Geometry check sheet. Reference: the model listing, model coordinates, mm. Face numbers are marked on the shaded views. A direction names the side the tool comes from. Round coordinates to 2 decimals unless told otherwise and drop trailing zeros. Order: outer loops, then holes, each group sorted by start corner. A loop starts at its lowest first (then second) coordinate and runs counter-clockwise, first axis right, second up.
(1) Material ranges on line 1 along Y through (x, z) = (16.5, 0.9); line 2 along Y through (x, z) = (-15.5, 0.25); line 3 along Z through (x, y) = (-14.5, 12), recorded low to high.
(2) Sectioned sample at A-A (z = -2.75). Record the boundary of the cut face in (x, y).
(3) Go/stop test with flat-tipped pins: pin 1 (2 mm diameter, centred on y = -2, z = -2.5, fed in from -X); pin 2 (1 mm diameter, centred on y = 1, z = -1, fed in from +X); pin 3 (1.2 mm diameter, centred on x = 19, z = -4, fed in from +Y). Record where each tip stops, or that it passes through.
(4) Sectioned sample at C-C (y = 9.4). Record the boundary of the cut face in (x, z).
(5) Release check for a two-part mould opening along X. For the marked faces 1 and 2 record: +X half, -X half, draft (parallel to the pull), parting line (faces both ways), or undercut.
(6) Set-up check for the marked faces 3 and 4: record each of +Z, -Z, +X, -X, +Y, -Y from which the full face is reachable in a straight line by a thin tool's end or side.
(7) Sectioned sample at B-B (x = 16.5). Record the boundary of the cut face in (y, z), plus the area to 4 significant figures.
(8) Sectioned sample at D-D (x = 4.5). Record the boundary of the cut face in (y, z).
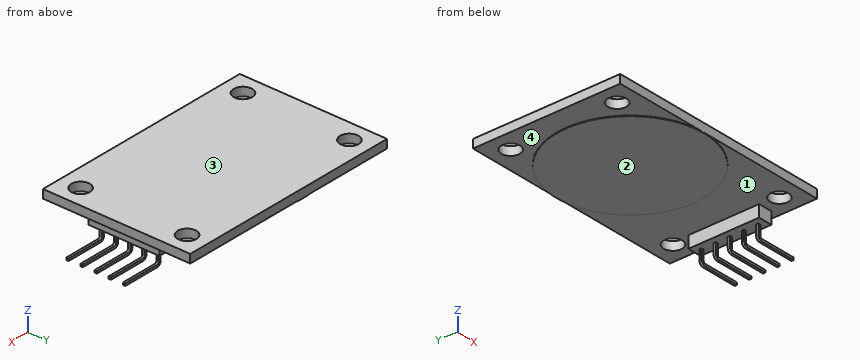
from build123d import *

# Parameters (mm, degrees)
SKETCH_1_W          = 40
SKETCH_1_H          = 26
EXTRUDE_1_DEPTH     = 1.5
SKETCH_2_R          = 1.65
CUT_EXTRUDE_1_DEPTH = 1.5
SKETCH_3_R          = 13
EXTRUDE_2_DEPTH     = 0.1
SKETCH_4_W          = 2.5
SKETCH_4_H          = 12.5
EXTRUDE_3_DEPTH     = 2.1
SKETCH_5_W          = 0.4
SKETCH_5_H          = 0.4


with BuildPart() as part:
    # 草图1 → 凸台-拉伸1 (new body)
    with BuildSketch(Plane.XY):
        Rectangle(SKETCH_1_W, SKETCH_1_H)
    extrude(amount=EXTRUDE_1_DEPTH)

    # 草图2 → 切除-拉伸1 (cut)
    with BuildSketch(Plane.XY.offset(1.5)):
        with Locations((-16.5, 9.4)):
            Circle(SKETCH_2_R)
        with Locations((16.5, 9.4)):
            Circle(SKETCH_2_R)
        with Locations((16.5, -9.4)):
            Circle(SKETCH_2_R)
        with Locations((-16.5, -9.4)):
            Circle(SKETCH_2_R)
    extrude(amount=-CUT_EXTRUDE_1_DEPTH, mode=Mode.SUBTRACT)

    # 草图3 → 凸台-拉伸2 (add)
    with BuildSketch(Plane(origin=(0, 0, 0), x_dir=(-1, 0, 0), z_dir=(0, 0, -1))):
        with Locations(Location((3, 0, 0), (0, 0, 270))):
            Circle(SKETCH_3_R)
    extrude(amount=EXTRUDE_2_DEPTH)

    # 草图4 → 凸台-拉伸3 (add)
    with BuildSketch(Plane(origin=(0, 0, 0), x_dir=(-1, 0, 0), z_dir=(0, 0, -1))):
        with Locations((-17.25, 0)):
            Rectangle(SKETCH_4_W, SKETCH_4_H)
    extrude(amount=EXTRUDE_3_DEPTH)

    # 扫描1: sweep along a path in 草图6
    with BuildLine(Plane(origin=(0, 5.2, 0), x_dir=(-1, 0, 0), z_dir=(0, -1, 0))) as sweep_1_path:
        Line((-17.25, 2.1), (-17.25, 3.9))
        ThreePointArc((-17.25, 3.9), (-17.396446609, 4.253553391), (-17.75, 4.4))
        Line((-17.75, 4.4), (-24.25, 4.4))
    # 草图5 → 扫描1 (sweep)
    with BuildSketch(Plane(origin=(0, 0, -2.1), x_dir=(-1, 0, 0), z_dir=(0, 0, -1))):
        with Locations((-17.25, 2.5)):
            Rectangle(SKETCH_5_W, SKETCH_5_H)
        with Locations((-17.25, 5)):
            Rectangle(SKETCH_5_W, SKETCH_5_H)
        with Locations((-17.25, 0)):
            Rectangle(SKETCH_5_W, SKETCH_5_H)
        with Locations((-17.25, -2.5)):
            Rectangle(SKETCH_5_W, SKETCH_5_H)
        with Locations((-17.25, -5)):
            Rectangle(SKETCH_5_W, SKETCH_5_H)
    sweep(path=sweep_1_path.line)


solid = part.part
Answer below:
1. line 1: y = -13 to -11.05, -7.75 to 7.75, 11.05 to 13
1. line 2: y = -13 to -10.71, -8.09 to 8.09, 10.71 to 13
1. line 3: z = 0 to 1.5
2. outline: (17.05, -5.2) - (17.45, -5.2) - (17.45, -4.8) - (17.05, -4.8) - close; (17.05, -2.7) - (17.45, -2.7) - (17.45, -2.3) - (17.05, -2.3) - close; (17.05, -0.2) - (17.45, -0.2) - (17.45, 0.2) - (17.05, 0.2) - close; (17.05, 2.3) - (17.45, 2.3) - (17.45, 2.7) - (17.05, 2.7) - close; (17.05, 4.8) - (17.45, 4.8) - (17.45, 5.2) - (17.05, 5.2) - close
3. pin 1: stops at x = 16
3. pin 2: stops at x = 18.5
3. pin 3: stops at y = 5.2
4. outline: (-20, 0) - (-18.15, 0) - (-18.15, 1.5) - (-20, 1.5) - close; (-14.85, 0) - (-11.98, 0) - (-11.98, -0.1) - (5.98, -0.1) - (5.98, 0) - (14.85, 0) - (14.85, 1.5) - (-14.85, 1.5) - close; (18.15, 0) - (20, 0) - (20, 1.5) - (18.15, 1.5) - close
5. face 1: undercut
5. face 2: draft
6. face 3: +Z, +X, -X, +Y, -Y
6. face 4: -Z, -X
7. outline: (-13, 0) - (-11.05, 0) - (-11.05, 1.5) - (-13, 1.5) - close; (-7.75, 0) - (-6.25, 0) - (-6.25, -2.1) - (6.25, -2.1) - (6.25, 0) - (7.75, 0) - (7.75, 1.5) - (-7.75, 1.5) - close; (11.05, 0) - (13, 0) - (13, 1.5) - (11.05, 1.5) - close
7. area: 55.35 mm2
8. outline: (-13, 0) - (-10.62, 0) - (-10.62, -0.1) - (10.62, -0.1) - (10.62, 0) - (13, 0) - (13, 1.5) - (-13, 1.5) - close
